Work out the finished part from the listing and answer in its coordinate system (mm). Give positions to 0.01 mm unless a question says otherwise; leave off trailing zeros. Order: outer loops, then holes, each group sorted by start corner. A loop starts at its lowest first (then second) coordinate and runs counter-clockwise, first axis right, second up. Notation, with made-up numbers: (37, -1.5) - (45, -1.5) arc R20 cw to (45, 8.5) - close; hole circle Ø4 at (-39, 0.25). An arc over 180 degrees is marked (long way). Write each question's results on one line, items separated by ' | '.
from build123d import *

# Parameters (mm, degrees)
F1_DEPTH = 1.25
F2_DEPTH = 0.5
F3_DEPTH = 0.5
F4_T     = -0.1
F6_DEPTH = 0.1
F8_DEPTH = 0.1
F9_D     = 2
F11_D    = 0.3


with BuildPart() as f1:
    # F0 (on Right) → F1 (new body, symmetric)
    with BuildSketch(Plane.YZ):
        Polygon((-96.8298226595, 19.8576506227), (-96.8298226595, 24.8576506227), (-121.8298226595, 24.8576506227), (-121.8298226595, 19.8576506227), (-114.4798226595, 19.8576506227), (-114.3298226595, 19.8576506227), (-114.2798226595, 19.8576506227), (-109.2798226595, 19.8576506227), (-104.2298226595, 19.8576506227), (-104.0798226595, 19.8576506227), align=None)
    extrude(amount=F1_DEPTH, both=True)

    # F0 (on Right) → F2 (join)
    with BuildSketch(Plane.YZ):
        with BuildLine():
            ThreePointArc((-109.0798226595, 14.8576506227), (-107.6153565654, 18.3931845287), (-104.0798226595, 19.8576506227))
            Line((-104.0798226595, 19.8576506227), (-104.2298226595, 19.8576506227))
            Line((-104.2298226595, 19.8576506227), (-109.2798226595, 19.8576506227))
            Line((-109.2798226595, 19.8576506227), (-109.2798226595, 9.8576506227))
            Line((-109.2798226595, 9.8576506227), (-109.0798226595, 9.8576506227))
            Line((-109.0798226595, 9.8576506227), (-109.0798226595, 14.8576506227))
        make_face()
        with BuildLine():
            Line((-114.3298226595, 19.8576506227), (-114.4798226595, 19.8576506227))
            ThreePointArc((-114.4798226595, 19.8576506227), (-110.9442887536, 18.3931845287), (-109.4798226595, 14.8576506227))
            Line((-109.4798226595, 14.8576506227), (-109.4798226595, 9.8576506227))
            Line((-109.4798226595, 9.8576506227), (-109.2798226595, 9.8576506227))
            Line((-109.2798226595, 9.8576506227), (-109.2798226595, 19.8576506227))
            Line((-109.2798226595, 19.8576506227), (-114.2798226595, 19.8576506227))
            Line((-114.2798226595, 19.8576506227), (-114.3298226595, 19.8576506227))
        make_face()
    extrude(amount=F2_DEPTH)

    # F0 (on Right) → F3 (join)
    with BuildSketch(Plane.YZ):
        with BuildLine():
            ThreePointArc((-109.0798226595, 14.8576506227), (-107.6153565654, 18.3931845287), (-104.0798226595, 19.8576506227))
            Line((-104.0798226595, 19.8576506227), (-104.2298226595, 19.8576506227))
            Line((-104.2298226595, 19.8576506227), (-109.2798226595, 19.8576506227))
            Line((-109.2798226595, 19.8576506227), (-109.2798226595, 9.8576506227))
            Line((-109.2798226595, 9.8576506227), (-109.0798226595, 9.8576506227))
            Line((-109.0798226595, 9.8576506227), (-109.0798226595, 14.8576506227))
        make_face()
        with BuildLine():
            Line((-114.3298226595, 19.8576506227), (-114.4798226595, 19.8576506227))
            ThreePointArc((-114.4798226595, 19.8576506227), (-110.9442887536, 18.3931845287), (-109.4798226595, 14.8576506227))
            Line((-109.4798226595, 14.8576506227), (-109.4798226595, 9.8576506227))
            Line((-109.4798226595, 9.8576506227), (-109.2798226595, 9.8576506227))
            Line((-109.2798226595, 9.8576506227), (-109.2798226595, 19.8576506227))
            Line((-109.2798226595, 19.8576506227), (-114.2798226595, 19.8576506227))
            Line((-114.2798226595, 19.8576506227), (-114.3298226595, 19.8576506227))
        make_face()
    extrude(amount=-F3_DEPTH)

    # F4
    f4_openings = [f1.faces().sort_by_distance(p)[0] for p in [
        (0, -96.829823, 22.357651),
        (0, -121.829823, 22.357651),
    ]]
    offset(amount=F4_T, openings=f4_openings, kind=Kind.INTERSECTION)

    # F5 (on face) → F6 (join)
    with BuildSketch(Plane.XZ.offset(121.8298226595)):
        Polygon((0, 24.7576506227), (-1.15, 24.7576506227), (-1.15, 19.9576506227), (0, 19.9576506227), (0, 22.4076506227), align=None)
        Polygon((1.15, 24.7576506227), (0, 24.7576506227), (0, 22.4076506227), (0, 19.9576506227), (1.15, 19.9576506227), align=None)
    extrude(amount=-F6_DEPTH)

    # F7 (on face) → F8 (join)
    with BuildSketch(Plane(origin=(0, -96.8298226595, 0), x_dir=(-1, 0, 0), z_dir=(0, 1, 0))):
        Polygon((0, 24.7576506227), (-1.15, 24.7576506227), (-1.15, 19.9576506227), (0, 19.9576506227), (0, 22.3576506227), align=None)
        Polygon((1.15, 24.7576506227), (0, 24.7576506227), (0, 22.3576506227), (0, 19.9576506227), (1.15, 19.9576506227), align=None)
    extrude(amount=-F8_DEPTH)

    # F9 (through all)
    with Locations(Plane(origin=(0, -96.8298226595, 0), x_dir=(-1, 0, 0), z_dir=(0, 1, 0))):
        with Locations((0, 22.3576506227)):
            Hole(F9_D / 2)

    # F11 (through all)
    with Locations(Plane(origin=(0, 0, 9.8576506227), x_dir=(1, 0, 0), z_dir=(0, 0, -1))):
        with Locations((0, 109.2798226595)):
            Hole(F11_D / 2)


solid = f1.part
1. A cutting plane is placed at B-B, the plane z = 20.75. Write down the section's boundary in (x, y).
Answer list:
outline: (-1.25, -121.83) - (1.25, -121.83) - (1.25, -96.83) - (-1.25, -96.83) - close; hole (-1.15, -121.73) - (1.15, -121.73) - (1.15, -96.93) - (-1.15, -96.93) - close
2. Given P1, Ø0.8, axis at x = 0, z = 12.5, coming from the -Y side; P2, Ø8, axis at y = -108.5, z = 16, coming from the -X side; P3, Ø0.8, axis at x = 0, z = 12.5, coming from the +Y side; P4, Ø1, axis at y = -101.5, z = 18, coming from the +X side, each flat-ended and moving along its own axis, determine where each tip first touches the part or whether it passes through.
Answer list:
P1: y = -109.48 | P2: x = -1.25 | P3: y = -109.08 | P4: through
3. A cutting plane is placed at C-C, the plane z = 13. Write down the section's boundary in (x, y), then the cut area to 3 significant figures.
Answer list:
outline: (-0.5, -109.48) - (0.5, -109.48) - (0.5, -109.08) - (-0.5, -109.08) - close; hole (-0.4, -109.38) - (-0.11, -109.38) arc R0.15 ccw to (0.11, -109.38) - (0.4, -109.38) - (0.4, -109.18) - (0.11, -109.18) arc R0.15 ccw to (-0.11, -109.18) - (-0.4, -109.18) - close | area: 0.225 mm^2
4. A cutting plane is placed at A-A, the plane y = -117.5. Write down the section's boundary in (x, z).
Answer list:
outline: (-1.25, 19.86) - (1.25, 19.86) - (1.25, 24.86) - (-1.25, 24.86) - close; hole (-1.15, 19.96) - (1.15, 19.96) - (1.15, 24.76) - (-1.15, 24.76) - close
5. A cutting plane is placed at D-D, the plane y = -107.5. Write down the section's boundary in (x, z), then the cut area to 3 significant figures.
Answer list:
outline: (-1.25, 19.86) - (-0.5, 19.86) - (-0.5, 18.5) - (0.5, 18.5) - (0.5, 19.86) - (1.25, 19.86) - (1.25, 24.86) - (-1.25, 24.86) - close; hole (-1.15, 19.96) - (-0.4, 19.96) - (-0.4, 18.64) - (0.4, 18.64) - (0.4, 19.96) - (1.15, 19.96) - (1.15, 24.76) - (-1.15, 24.76) - close | area: 1.76 mm^2
